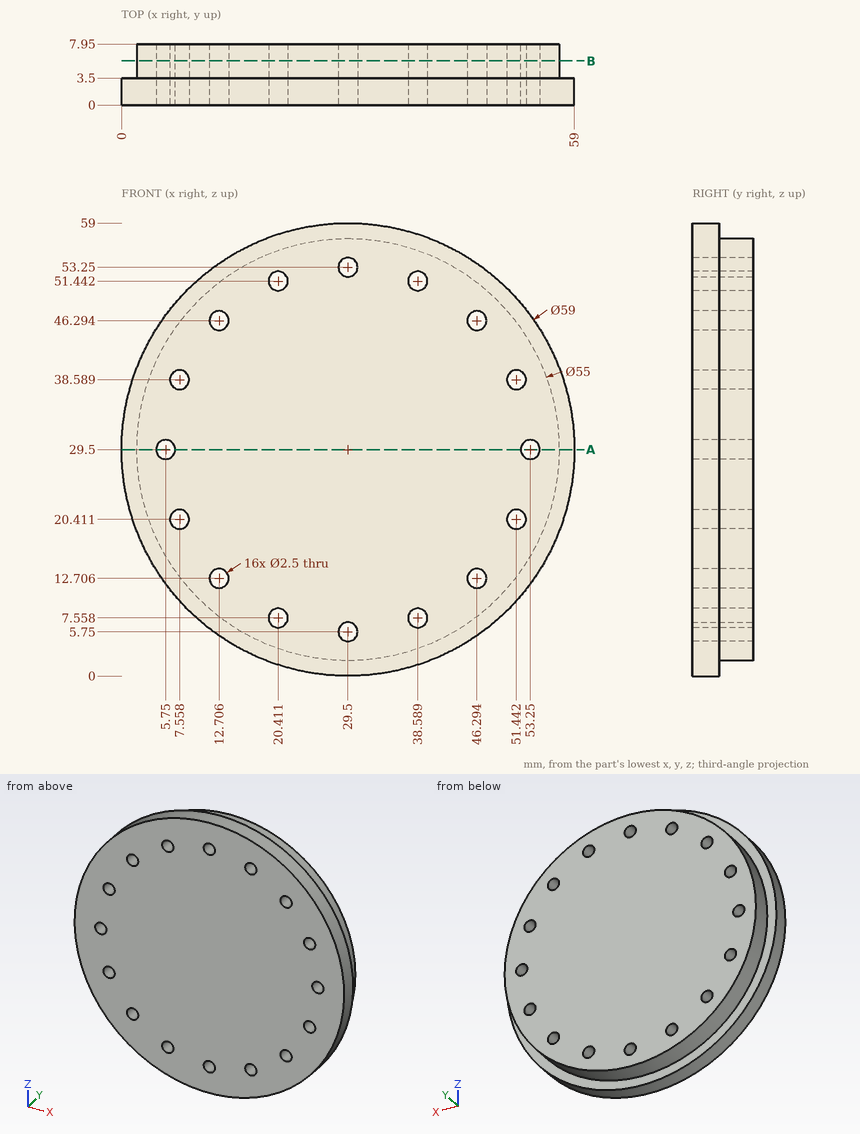
The figure shows three views and two pictorial views of one solid part (mm, origin at its lowest corner). Answer the questions. Give positions to 0.01 mm unless a question says otherwise; leave off trailing zeros. Write each loop counter-clockwise with the first axis right and the second up, starting at its lowest first coordinate (ties: lowest second). Pieces come first, ordered by that corner, then holes. Notation, with made-up numbers: M 53,63.25 L 68,63.25 A28 cw 68,102.25 Z; hole C 62,-37 d3. An arc over 180 degrees is marked long. One line per item, written item: value. Start each with the question number.
(1) Flat-ended cylindrical pins translate along their axes: pin 1 Ø1 at (x, y) = (15, 3) entering from -Z; pin 2 Ø3 at (x, z) = (46.29, 46.29) entering from -Y; pin 3 Ø3 at (y, z) = (5.5, 43.5) entering from -X (1 decimal); pin 4 Ø1 at (x, y) = (13.5, 1.5) entering from -Z. Find the tip coordinate at first contact, or state that the pin passes through.
(2) Find section B-B (y = 5.75). Give the number of separate pieces and of enclosed holes in the cut face, plus the area to 3 significant figures.
(3) Find the intervals of material crossed by line 1 (Z direction, x = 20, y = 1); line 2 (Z direction, x = 13.5, y = 2.5) (1 decimal); line 3 (X direction, y = 4.5, z = 30) (1 decimal), in increasing order.
(4) Find section A-A (z = 29.5). Determine the outline of the cut face in (x, y).
Results below:
1. pin 1: stops at z = 3.53
1. pin 2: stops at y = 0
1. pin 3: stops at x = 5
1. pin 4: stops at z = 4.4
2. separate pieces: 1
2. enclosed holes: 16
2. area: 2,300 mm^2
3. line 1: z = 1.57 to 6.38, 8.74 to 50.26, 52.62 to 57.43
3. line 2: z = 4.7 to 11.7, 13.7 to 45.3, 47.3 to 54.3
3. line 3: x = 2 to 4.6, 6.9 to 52.1, 54.4 to 57
4. outline: M 0,0 L 4.5,0 L 4.5,7.95 L 2,7.95 L 2,3.5 L 0,3.5 Z; M 7,0 L 52,0 L 52,7.95 L 7,7.95 Z; M 54.5,0 L 59,0 L 59,3.5 L 57,3.5 L 57,7.95 L 54.5,7.95 Z
